Source: CAD feature listing. Evaluate the final solid. Frame: model axes, mm. Face numbers are marked on the shaded views. A direction names the side the tool comes from. Round coordinates to 2 decimals unless told otherwise and drop trailing zeros. Order: outer loops, then holes, each group sorted by start corner. A loop starts at its lowest first (then second) coordinate and runs counter-clockwise, first axis right, second up. Notation, with made-up numbers: (87.25, 75) -> (129.25, 75) arc R8 ccw to (129.25, 84) -> close; hole circle Ø9 at (21.5, 52.25). An arc over 180 degrees is marked (long way). Use a Markdown table: item, result. Add a question column.
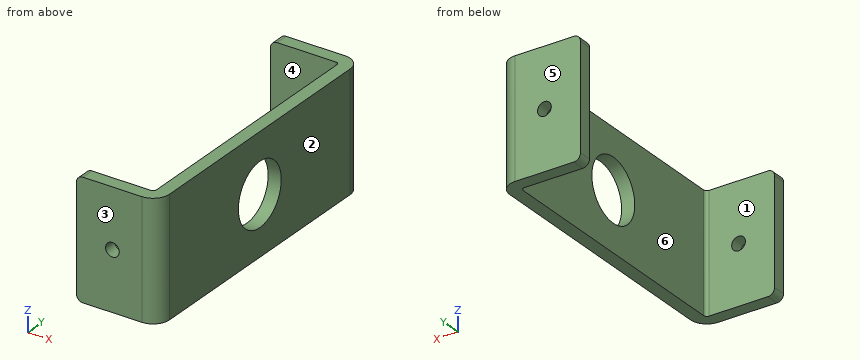
```python
from build123d import *

# Parameters (mm, degrees)
BASE_FLANGE1_START    = -18
BASE_FLANGE1_DEPTH    = 36
FILLET1_R             = 2
M5_TAPPED_HOLE1_D     = 4.2
M5_TAPPED_HOLE1_DEPTH = 4
SKETCH8_R             = 9.5
CUT_EXTRUDE1_DEPTH    = 55.534392818


# Read off the part's stored shape, not the designer's step: Base-Flange1
with BuildPart() as part:
    # Base-Flange1 outline → Base-Flange1 (new body)
    with BuildSketch(Plane.XY.offset(BASE_FLANGE1_START)):
        with BuildLine():
            Line((-5, 45), (-25, 45))
            Line((-25, 45), (-25, 41))
            Line((-25, 41), (-5, 41))
            ThreePointArc((-5, 41), (-4.292893219, 40.707106781), (-4, 40))
            Line((-4, 40), (-4, -40))
            ThreePointArc((-4, -40), (-4.292893219, -40.707106781), (-5, -41))
            Line((-5, -41), (-25, -41))
            Line((-25, -41), (-25, -45))
            Line((-25, -45), (-5, -45))
            ThreePointArc((-5, -45), (-1.464466094, -43.535533906), (0, -40))
            Line((0, -40), (0, 40))
            ThreePointArc((0, 40), (-1.464466094, 43.535533906), (-5, 45))
        make_face()
    extrude(amount=BASE_FLANGE1_DEPTH)

    # Fillet1
    fillet1_edges = [part.edges().sort_by_distance(p)[0] for p in [
        (-25, -43, -18),
        (-25, 43, -18),
        (-25, -43, 18),
        (-25, 43, 18),
    ]]
    fillet(fillet1_edges, radius=FILLET1_R)

    # M5 Tapped Hole1
    with Locations(Plane(origin=(0, 45, 0), x_dir=(1, 0, 0), z_dir=(0, 1, 0))):
        with Locations((-14, 0)):
            m5_tapped_hole1 = Hole(M5_TAPPED_HOLE1_D / 2, depth=M5_TAPPED_HOLE1_DEPTH)

    # Mirror1: M5 Tapped Hole1 across plane
    add(m5_tapped_hole1.mirror(Plane.ZX), mode=Mode.SUBTRACT)

    # Sketch8 → Cut-Extrude1 (cut, through all)
    with BuildSketch(Plane(origin=(0, 0, 0), x_dir=(0, 0, -1), z_dir=(1, 0, 0))):
        with Locations(Location((0, 0, 0), (0, 0, 90))):
            Circle(SKETCH8_R)
    extrude(amount=-CUT_EXTRUDE1_DEPTH, mode=Mode.SUBTRACT)


solid = part.part
```
1) Section A-A on x = -14. Output: boundary loops of the cut face in (y, z).
2) Section D-D on x = -18.5. Output: boundary loops of the cut face in (y, z), then the cut area to 3 significant figures.
3) First-contact query: pin 1 Ø15 at (y, z) = (0, 0) entering from -X; pin 2 Ø6 at (y, z) = (21, -4.5) entering from -X. Flat tips, straight axial feed; report the tip coordinate or a pass-through.
4) Draft query along Y for the marked faces 3, 4, 5 and 6. Return one class per face: pulls with the +Y half, pulls with the -Y half, needs draft (parallel to the pull), parting line crosses it, or undercut.
5) Section C-C on z = 0. Output: boundary loops of the cut face in (x, y).
6) Section B-B on y = 0. Output: boundary loops of the cut face in (x, z).
7) Line query: probe 1 along Z at (x, y) = (-14, 43.55); probe 2 along Z at (x, y) = (-2.4, 0); probe 3 along Y at (x, z) = (-5, -5.5). Output: solid intervals per line, ascending. Write a range as from..to.
8) Reachability of the marked faces 1 and 2 from +Z, -Z, +X, -X, +Y, -Y: full face, straight path, thin tool, end or side. Return the list, or none.
Conclusion:
| question | item | result |
|---|---|---|
| 1 | outline | (-45, -18) -> (-41, -18) -> (-41, -2.1) -> (-45, -2.1) -> close; (-45, 2.1) -> (-41, 2.1) -> (-41, 18) -> (-45, 18) -> close; (41, -18) -> (45, -18) -> (45, -2.1) -> (41, -2.1) -> close; (41, 2.1) -> (45, 2.1) -> (45, 18) -> (41, 18) -> close |
| 2 | outline | (-45, -18) -> (-41, -18) -> (-41, 18) -> (-45, 18) -> close; (41, -18) -> (45, -18) -> (45, 18) -> (41, 18) -> close |
| 2 | area | 288 mm^2 |
| 3 | pin 1 | passes through |
| 3 | pin 2 | stops at x = -4 |
| 4 | face 3 | pulls with the -Y half |
| 4 | face 4 | undercut |
| 4 | face 5 | pulls with the +Y half |
| 4 | face 6 | undercut |
| 5 | outline | (-25, -45) -> (-16.1, -45) -> (-16.1, -41) -> (-25, -41) -> close; (-25, 41) -> (-16.1, 41) -> (-16.1, 45) -> (-25, 45) -> close; (-11.9, -45) -> (-5, -45) arc R5 ccw to (0, -40) -> (0, -9.5) -> (-4, -9.5) -> (-4, -40) arc R1 cw to (-5, -41) -> (-11.9, -41) -> close; (-11.9, 41) -> (-5, 41) arc R1 cw to (-4, 40) -> (-4, 9.5) -> (0, 9.5) -> (0, 40) arc R5 ccw to (-5, 45) -> (-11.9, 45) -> close |
| 6 | outline | (-4, -18) -> (0, -18) -> (0, -9.5) -> (-4, -9.5) -> close; (-4, 9.5) -> (0, 9.5) -> (0, 18) -> (-4, 18) -> close |
| 7 | probe 1 | z = -18..-2.1, 2.1..18 |
| 7 | probe 2 | z = -18..-9.5, 9.5..18 |
| 7 | probe 3 | y = -45..-41, 41..45 |
| 8 | face 1 | +Z, -Z, -X |
| 8 | face 2 | +Z, -Z, +X, +Y, -Y |
